Work out the finished part from the listing and answer in its coordinate system (mm). A direction names the side the tool comes from. Round coordinates to 2 decimals unless told otherwise and drop trailing zeros. Order: outer loops, then holes, each group sorted by start corner. A loop starts at its lowest first (then second) coordinate and runs counter-clockwise, first axis right, second up. Notation, with made-up numbers: (42, 75) -> (93, 75) arc R22 ccw to (93, 92) -> close; hole circle Ø7 at (3.5, 39.5). An arc over 180 degrees is marked (long way). Use a Markdown table: item, result. Add a question column.
Item 1: A tool of negligible diameter and unlimited length cuts with its end or side. For faces 4 (the flat face through (77, 0, 31.621)), 5 (the flat face through (1, 34, 19.752)), 6 (the flat face through (1, -22, 19.752)), 7 (the flat face through (51, 20, 42.632)), 8 (the flat face through (56, 23, 58.639)), from which of +Z, -Z, +X, -X, +Y, -Y can it reach the whole face along a straight path? Write none if from no direction.
Item 2: A cutting plane is placed at B-B, the plane y = -22. Determine the outline of the cut face in (x, z) (1 decimal), plus the area to 3 significant figures.
Item 3: A cutting plane is placed at C-C, the plane x = 79. Determine the outline of the cut face in (y, z).
Item 4: Flat-ended cylindrical pins translate along their axes: P1, Ø18, axis at x = 90.5, y = 2.5, coming from the +Z side; P2, Ø2, axis at x = -8.5, z = 55.5, coming from the -Y side; P3, Ø8.5, axis at x = 54.5, y = 14.5, coming from the -Z side. Find the tip coordinate at first contact, or state that the pin passes through.
Item 5: Find the intervals of material crossed by L1, parallel to Z at x = -25.5, y = 42.5; L2, parallel to Z at x = 99, y = 3; L3, parallel to Y at x = 77, z = 46.5, in increasing order. Write a range as [from, to].
Item 6: A cutting plane is placed at A-A, the plane z = -5. Determine the outline of the cut face in (x, y) (3 decimals), plus the area to 3 significant figures.
Item 7: A cutting plane is placed at D-D, the plane y = -5. Determine the outline of the cut face in (x, z) (1 decimal), plus the area to 3 significant figures.
Item 8: For a pull along X with two mould halves and no side action, classify faces 1 (the cylindrical face through (36.53, -43.44, -2.3)), 2 (the conical face through (-34.29, 41.24, 17.81)), 3 (the flat face through (51, -20, 42.632)) as +X half, -X half, draft (parallel to the pull), parting line (faces both ways), or undercut.
from build123d import *

# Parameters (mm, degrees)
F1_DEPTH     = 48.44446
F0_W         = 21.137111498
F0_H         = 16.0069091111
F2_DEPTH     = 24.04666
F3_DEPTH     = 24.04666
F4_DEPTH     = 15.49987
F5_DEPTH     = 16.86318
F7_R         = 16.6410292326
F8_T1_DEPTH  = 49.2679415348
F8_T3_DEPTH  = 7.7567707674
F8_T5_DEPTH  = 31.8034307674
F8_T7_DEPTH  = 7.7567707674
F8_T10_ANGLE = 90
F8_T12_ANGLE = 90
F8_T14_ANGLE = 90
F8_T16_ANGLE = 90


# Not quite as in the source:
# - a fillet or chamfer that OpenCascade refuses, or shapes differently, is made with other operations: its cross-section is extruded or revolved along the edge and cut away or added


with BuildPart() as f1:
    # F0 (on Front) → F1 (new body, symmetric)
    with BuildSketch(Plane.XZ):
        Polygon((-41.275, -19.751769717), (41.275, -19.751769717), (41.275, 19.751769717), (25.2680908889, 19.751769717), (-41.275, 19.751769717), align=None)
    extrude(amount=F1_DEPTH, both=True)

    # F0 (on Front) → F2 (join, symmetric)
    with BuildSketch(Plane.XZ):
        with BuildLine():
            Line((25.2680908889, 19.751769717), (41.275, 19.751769717))
            Line((41.275, 19.751769717), (41.275, 36.7465044527))
            ThreePointArc((41.275, 36.7465044527), (43.3382033754, 41.2513095059), (48.0968345152, 42.6317103213))
            Line((48.0968345152, 42.6317103213), (55.0704259122, 42.6317103213))
            Line((55.0704259122, 42.6317103213), (55.0704259122, 58.6386194325))
            Line((55.0704259122, 58.6386194325), (48.9036156195, 58.6386194325))
            ThreePointArc((48.9036156195, 58.6386194325), (32.3044367766, 52.8547533301), (25.2680908889, 36.7465044527))
            Line((25.2680908889, 36.7465044527), (25.2680908889, 19.751769717))
        make_face()
        with Locations((65.6389816612, 50.6351648769)):
            Rectangle(F0_W, F0_H)
        Polygon((76.2075374102, 64.215389511), (76.2075374102, 58.6386194325), (76.2075374102, 42.6317103213), (76.2075374102, 31.6205449668), (105.8704259122, 31.6205449668), (105.8704259122, 64.215389511), align=None)
    extrude(amount=F2_DEPTH, both=True)

    # F0 (on Front) → F3 (join, through all)
    with BuildSketch(Plane.XZ):
        with BuildLine():
            add(Edge.make_bspline(
                [(-41.275, 19.751769717), (-42.804622746, 65.2502314703), (54.8739225948, 71.3754703993), (55.0704259122, 58.7153048291)],
                knots=[0, 0, 0, 0, 103.688468472, 103.688468472, 103.688468472, 103.688468472], degree=3))
            Line((-41.275, 19.751769717), (25.2680908889, 19.751769717))
            Line((25.2680908889, 19.751769717), (25.2680908889, 36.7465044527))
            ThreePointArc((25.2680908889, 36.7465044527), (32.3044367766, 52.8547533301), (48.9036156195, 58.6386194325))
            Line((48.9036156195, 58.6386194325), (55.0704259122, 58.6386194325))
            Line((55.0704259122, 58.6386194325), (55.0704259122, 58.7153048291))
        make_face()
    extrude(amount=-F3_DEPTH)

    # F4 (add): a face of the model
    f4_faces = [f1.faces().sort_by_distance(p)[0] for p in [
        (105.8704259122, 0, 47.9179672389),
    ]]
    extrude(f4_faces, amount=-F4_DEPTH)

    # F5 (cut): a face of the model
    f5_faces = [f1.faces().sort_by_distance(p)[0] for p in [
        (105.8704259122, 0, 47.9179672389),
    ]]
    extrude(f5_faces, amount=-F5_DEPTH, mode=Mode.SUBTRACT)

    # F0 (on Front) → F6 (revolve)
    with BuildSketch(Plane.XZ):
        Polygon((76.2075374102, 64.215389511), (76.2075374102, 58.6386194325), (76.2075374102, 42.6317103213), (76.2075374102, 31.6205449668), (105.8704259122, 31.6205449668), (105.8704259122, 64.215389511), align=None)
    revolve(axis=Axis((76.2075374102, 0, 47.9179672389), (0, 0, 1)))

    # F7
    f7_edges = [f1.edges().sort_by_distance(p)[0] for p in [
        (-41.275, -48.44446, 0),
        (41.275, -48.44446, 0),
        (41.275, 48.44446, 0),
        (-41.275, 48.44446, 0),
    ]]
    fillet(f7_edges, radius=F7_R)

    # F8: chamfer of 5.08 on 2 edges, made by hand

    # F8_s2 → F8_t1 (cut)
    with BuildSketch(Plane.YZ.offset(-24.6339707674)):
        Polygon((43.36446, 19.751769717), (48.44446, 14.671769717), (48.44446, 19.751769717), align=None)
        Polygon((-43.36446, 19.751769717), (-48.44446, 14.671769717), (-48.44446, 19.751769717), align=None)
    extrude(amount=F8_T1_DEPTH, mode=Mode.SUBTRACT)

    # F8_s4 → F8_t3 (cut)
    with BuildSketch(Plane.XZ.offset(24.04666)):
        Polygon((36.195, 19.751769717), (41.275, 14.671769717), (41.275, 19.751769717), align=None)
    extrude(amount=F8_T3_DEPTH, mode=Mode.SUBTRACT)

    # F8_s6 → F8_t5 (cut)
    with BuildSketch(Plane.XZ):
        Polygon((-41.275, 14.671769717), (-36.195, 19.751769717), (-41.275, 19.751769717), align=None)
    extrude(amount=F8_T5_DEPTH, mode=Mode.SUBTRACT)

    # F8_s8 → F8_t7 (cut)
    with BuildSketch(Plane.XZ.offset(-31.8034307674)):
        Polygon((-41.275, 14.671769717), (-36.195, 19.751769717), (-41.275, 19.751769717), align=None)
        Polygon((36.195, 19.751769717), (41.275, 14.671769717), (41.275, 19.751769717), align=None)
    extrude(amount=F8_T7_DEPTH, mode=Mode.SUBTRACT)

    # F8_s9 → F8_t10 (revolve, cut)
    with BuildSketch(Plane.XZ.offset(31.8034307674)):
        Polygon((-41.275, 14.671769717), (-36.195, 19.751769717), (-41.275, 19.751769717), align=None)
    revolve(axis=Axis((-24.6339707674, -31.8034307674, 19.751769717), (0, 0, 1)), revolution_arc=F8_T10_ANGLE, mode=Mode.SUBTRACT)

    # F8_s11 → F8_t12 (revolve, cut)
    with BuildSketch(Plane.YZ.offset(24.6339707674)):
        Polygon((-43.36446, 19.751769717), (-48.44446, 14.671769717), (-48.44446, 19.751769717), align=None)
    revolve(axis=Axis((24.6339707674, -31.8034307674, 19.751769717), (0, 0, 1)), revolution_arc=F8_T12_ANGLE, mode=Mode.SUBTRACT)

    # F8_s13 → F8_t14 (revolve, cut)
    with BuildSketch(Plane.YZ.offset(24.6339707674)):
        Polygon((43.36446, 19.751769717), (48.44446, 14.671769717), (48.44446, 19.751769717), align=None)
    revolve(axis=Axis((24.6339707674, 31.8034307674, 19.751769717), (0, 0, -1)), revolution_arc=F8_T14_ANGLE, mode=Mode.SUBTRACT)

    # F8_s15 → F8_t16 (revolve, cut)
    with BuildSketch(Plane.XZ.offset(-31.8034307674)):
        Polygon((-41.275, 14.671769717), (-36.195, 19.751769717), (-41.275, 19.751769717), align=None)
    revolve(axis=Axis((-24.6339707674, 31.8034307674, 19.751769717), (0, 0, -1)), revolution_arc=F8_T16_ANGLE, mode=Mode.SUBTRACT)


solid = f1.part
Reported:
| question | item | result |
|---|---|---|
| 1 | face 4 | -Z, +X, +Y, -Y |
| 1 | face 5 | +Z, +X, -X, +Y |
| 1 | face 6 | +Z, -X, -Y |
| 1 | face 7 | -Z, +Y |
| 1 | face 8 | +Z, +Y |
| 2 | outline | (-41.3, -19.8) -> (41.3, -19.8) -> (41.3, 36.7) arc R5.9 cw to (48.1, 42.6) -> (56.3, 42.6) -> (56.3, 31.6) -> (96.1, 31.6) -> (96.1, 64.2) -> (56.3, 64.2) -> (56.3, 58.6) -> (48.9, 58.6) arc R22 ccw to (25.3, 36.7) -> (25.3, 19.8) -> (-36.2, 19.8) -> (-41.3, 14.7) -> close |
| 2 | area | 5,310 mm² |
| 3 | outline | (-29.53, 31.62) -> (29.53, 31.62) -> (29.53, 64.22) -> (-29.53, 64.22) -> close |
| 4 | P1 | z = 64.22 |
| 4 | P2 | y = 0 |
| 4 | P3 | z = 31.62 |
| 5 | L1 | [-19.75, 19.75] |
| 5 | L2 | [31.62, 64.22] |
| 5 | L3 | [-29.65, 29.65] |
| 6 | outline | (-41.275, -31.803) arc R16.641 ccw to (-24.634, -48.444) -> (24.634, -48.444) arc R16.641 ccw to (41.275, -31.803) -> (41.275, 31.803) arc R16.641 ccw to (24.634, 48.444) -> (-24.634, 48.444) arc R16.641 ccw to (-41.275, 31.803) -> close |
| 6 | area | 7,760 mm² |
| 7 | outline | (-41.3, -19.8) -> (41.3, -19.8) -> (41.3, 36.7) arc R5.9 cw to (47, 42.7) -> (47, 31.6) -> (105.4, 31.6) -> (105.4, 64.2) -> (47, 64.2) -> (47, 58.7) arc R22 ccw to (25.3, 36.7) -> (25.3, 19.8) -> (-36.2, 19.8) -> (-41.3, 14.7) -> close |
| 7 | area | 5,770 mm² |
| 8 | face 1 | +X half |
| 8 | face 2 | -X half |
| 8 | face 3 | undercut |
